Input: part model. Units: mm. Frame: model coordinates. A direction names the side the tool comes from. Coordinates: 2 decimals unless noted, no trailing zeros. Loops run counter-clockwise (first coordinate to the right, second up) from the corner with the lowest first, then second, coordinate; pieces in that order, holes last.
(1) Line query: L1, parallel to Z at x = 2, y = -1.5; L2, parallel to X at y = 6.5, z = 0; L3, parallel to Z at x = -3.25, y = -1.5. Output: solid intervals per line, ascending.
(2) Mould query, pull axis Z, two halves, no side actions, for faces 1 (the face through (0, -2, 2)), 2 (the face through (-0.1, 0, 3.4)), 3 (the face through (1.724, -2.049, -1.014)), 4 (the face through (-3, 6, 0)). Classes: released by +Z, released by -Z, zero draft, split by the parting line, or undercut.
(3) Set-up query: faces 5 (the face through (1.86, -3.26, -1.09)), 6 (the face through (0, 12, 0)). Return all of +Z, -Z, +X, -X, +Y, -Y with unobstructed straight access to the full face (end or side cutting, diameter ignored); none if empty.
(4) Section A-A, the plane y = 6. Return loops of the section in (x, z).
(5) Contact query for flat-ended pins moving along their axis: P1, Ø1.2, axis at x = -0.5, y = -2.5, coming from the -Z side; P2, Ø1, axis at x = 3, y = 3, coming from the -Z side; P3, Ø3, axis at x = 3, y = 7.5, coming from the -Z side. Output: stop coordinate, or through.
Solid Edge part; units mm, degrees
sketch "Sketch1" plane through (0, 0, 0) normal (0, 0, 1) x (1, 0, 0)
  line L0 (3, 0) -> (3, 12)
  line L1 (0, 12) -> (3, 12)
  line L2 (0, 0) -> (0, 12)
  line L3 (0, 0) -> (0, -3.3)
  line L4 (0, -3.3) -> (5.25, -3.3)
  line L5 (5.25, -3.3) -> (5.25, 0)
  line L6 (5.25, 0) -> (3, 0)
revolve "RevolvedProtrusion1" add sketch "Sketch1" angle 360 about axis through (0, 0, 0) along (0, 1, 0)
sketch "Sketch2" plane through (0, 0, 0) normal (1, 0, 0) x (0, 1, 0)
  line L0 (-3.3, 2.7915) -> (-1.22, 2.7915)
  line L1 (0.3917, 0) -> (-1.22, 2.7915)
  line L2 (-3.3, 0) -> (0.3917, 0)
  line L3 (-3.3, 0) -> (-3.3, 2.7915)
revolve "RevolvedCutout1" cut sketch "Sketch2" angle 360 about axis through (0, -4.5, 0) along (0, 1, 0)
sketch "Sketch3" plane through (0, -3.3, 0) normal (0, -1, 0) x (0, 0, 1)
  circle A0 centre (0, 0) radius 2.7915
  line L0 (-2, -1.1547) -> (0, -2.3094)
  line L1 (0, -2.3094) -> (2, -1.1547)
  line L2 (2, -1.1547) -> (2, 1.1547)
  line L3 (2, 1.1547) -> (0, 2.3094)
  line L4 (0, 2.3094) -> (-2, 1.1547)
  line L5 (-2, 1.1547) -> (-2, -1.1547)
extrude "Protrusion1" add sketch "Sketch3" against normal up to next
sketch "Sketch4" plane through (0, 0, 0) normal (0, 0, 1) x (1, 0, 0)
  line L0 (-2.3094, -3.3) -> (0, -3.3)
  line L1 (0, -3.3) -> (0, -2.6812)
  line L2 (0, -2.6812) -> (-2.3094, -3.3)
revolve "RevolvedCutout2" cut sketch "Sketch4" angle 360 about axis through (0, -4.5, 0) along (0, 1, 0)
fillet "Round1" radius 0.25 1 edges at (0, 0, -3)
chamfer "倒斜角_2" distance 0.4 angle 45 1 edges at (0, 12, -3)
cosmetic_thread "螺纹_3" thread depth 10
sketch "Sketch5" plane through (0, 0, 0) normal (0, 0, 1) x (1, 0, 0)
  arc A0 (-3.0553, -3.3) -> (-5.25, 0) centre (-1.6717, 0) cw
revolve "RevolvedCutout3" cut sketch "Sketch5" angle 360 about axis through (0, 0, 0) along (0, -1, 0) material side at (-4.6929, -2.0093, 0)
Report:
1. L1: z = -4.5 to -0.54, 0.54 to 4.5
1. L2: x = -3 to 3
1. L3: z = -3.69 to 3.69
2. face 1: undercut
2. face 2: zero draft
2. face 3: undercut
2. face 4: split by the parting line
3. face 5: -Y
3. face 6: +Z, -Z, +X, -X, +Y
4. outline: circle Ø6 at (0, 0)
5. P1: stops at z = -4.68
5. P2: stops at z = -1.66
5. P3: stops at z = -2.6
